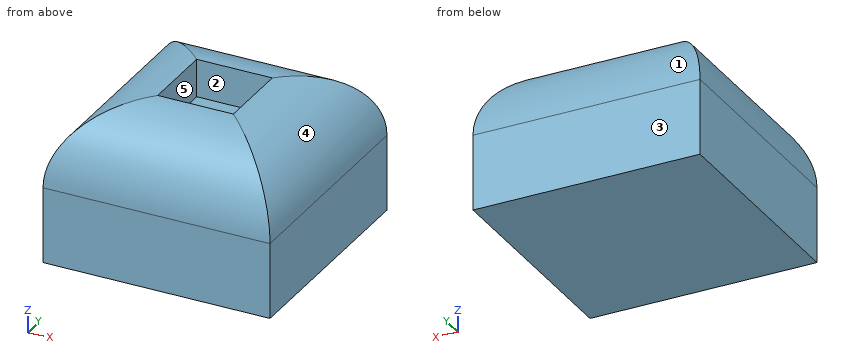
from build123d import *

# Parameters (mm, degrees)
F0_W     = 300
F0_H     = 300
F0_W_2   = 100
F0_H_2   = 100
F1_DEPTH = 200
F2_DEPTH = 150
F3_R     = 99.99999


# Not quite as in the source:
# - a fillet or chamfer is up to 0.001 mm smaller than in the source, because OpenCascade refuses the exact size


with BuildPart() as f1:
    # F0 (on Top) → F1 (new body)
    with BuildSketch(Plane.XY):
        Rectangle(F0_W, F0_H)
        Rectangle(F0_W_2, F0_H_2, mode=Mode.SUBTRACT)
    extrude(amount=F1_DEPTH)

    # F0 (on Top) → F2 (join)
    with BuildSketch(Plane.XY):
        Rectangle(F0_W_2, F0_H_2)
    extrude(amount=F2_DEPTH)

    # F3 (radius 100 in the source; OpenCascade refuses exactly that, so slightly less here)
    f3_edges = [f1.edges().sort_by_distance(p)[0] for p in [
        (-150, 0, 200),
        (0, -150, 200),
        (150, 0, 200),
        (0, 150, 200),
    ]]
    fillet(f3_edges, radius=F3_R)


solid = f1.part
Design review of the part built by this model. Coordinates are the model's own, in mm. Face numbers are marked on the shaded views. A direction names the side the tool comes from. Give positions to 0.01 mm unless a question says otherwise; leave off trailing zeros. Loops run counter-clockwise (first coordinate to the right, second up) from the corner with the lowest first, then second, coordinate; pieces in that order, holes last. Notation, with made-up numbers: (32.5, -5.75) -> (87.5, -5.75) arc R17 cw to (87.5, 26.25) -> close; hole circle Ø7 at (22, 32.25). An arc over 180 degrees is marked (long way). One line per question, with ' | ' between items. Start each with the question number.
(1) For the marked faces 1 and 2, list the 3-axis set-ups (+Z, -Z, +X, -X, +Y, -Y) from which the entire face can be reached by the end or side of a thin tool; tool diameter is ignored.
(2) Insertion check: P1, Ø15, axis at x = 21, z = 174.5, coming from the -Y side; P2, Ø8, axis at x = -44.5, z = 155.5, coming from the -Y side; P3, Ø12, axis at x = 41, y = -91.5, coming from the +Z side. Each pin has a flat end and moves straight along its axis. Give the tip position at first contact, or say it passes through.
(3) We need section D-D (y = 125). State the section outline as (x, z) points, and give its area (3 significant figures).
(4) For line 1 (Z direction, x = 24.5, y = -42.5); line 2 (Y direction, x = -6, z = 171); line 3 (X direction, y = -135, z = 103) (3 decimals), list the stretches that pass through material, from the lowest coordinate up.
(5) We need section C-C (z = 157). State the section outline as (x, y) points, and give its area (3 significant figures).
(6) Draft analysis for pull direction Y (two halves, no side actions). For the marked faces 3, 4 and 5, state which applies: +Y half, -Y half, draft (parallel to the pull), parting line (faces both ways), or undercut.
The answers:
1) face 1: +Z, +X, -X, +Y | face 2: +Z
2) P1: stops at y = -124.24 | P2: stops at y = -135.72 | P3: stops at z = 193.49
3) outline: (-150, 0) -> (150, 0) -> (150, 100) arc R100 ccw to (125, 166.14) -> (-125, 166.14) arc R100 ccw to (-150, 100) -> close | area: 48,800 mm^2
4) line 1: z = 0 to 150 | line 2: y = -120.42 to -50, 50 to 120.42 | line 3: x = -149.955 to 149.955
5) outline: (-132.16, -132.16) -> (132.16, -132.16) -> (132.16, 132.16) -> (-132.16, 132.16) -> close; hole (-50, -50) -> (50, -50) -> (50, 50) -> (-50, 50) -> close | area: 59,900 mm^2
6) face 3: +Y half | face 4: draft | face 5: undercut
